Model file for the job. Use its own axes, mm. Face numbers are marked on the shaded views. A direction names the side the tool comes from. Round coordinates to 2 decimals unless told otherwise and drop trailing zeros. Loops run counter-clockwise (first coordinate to the right, second up) from the corner with the lowest first, then second, coordinate; pieces in that order, holes last. Notation, with made-up numbers: (2, 50) -> (20, 50) arc R34 cw to (20, 80) -> close; hole circle Ø6 at (37.25, 63.25). An arc over 180 degrees is marked (long way). Use a Markdown table: item, result.
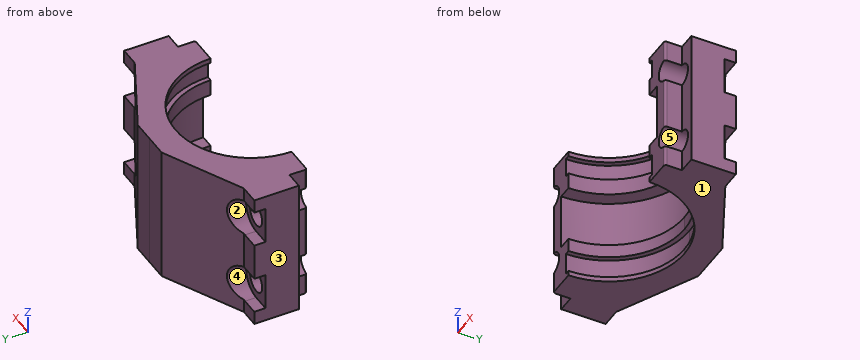
from build123d import *

# Parameters (mm, degrees)
BOSS_EXTRUDE1_DEPTH     = 56
SKETCH2_W               = 2
SKETCH2_H               = 7.81
SKETCH2_W_2             = 5.5
SKETCH2_H_2             = 23
SKETCH2_W_3             = 1.997029369
SKETCH2_H_3             = 9
CUT_EXTRUDE1_DEPTH      = 79.498407627
CUT_EXTRUDE1_DEPTH_BACK = 4.5
SKETCH5_R               = 4.5
CUT_EXTRUDE2_DEPTH      = 78.183223566


with BuildPart() as part:
    # Sketch1 → Boss-Extrude1 (new body)
    with BuildSketch(Plane.XY):
        with BuildLine():
            Line((-30.5, 0), (-41, 0))
            ThreePointArc((-41, 0), (-41.707106781, 0.292893219), (-42, 1))
            Line((-42, 1), (-42, 7))
            Line((-42, 7), (-49, 7))
            Line((-49, 7), (-49, 25))
            Line((-49, 25), (-41.09, 25))
            Line((-41.09, 25), (-9, 41))
            Line((-9, 41), (0, 41))
            Line((0, 41), (0, 30.5))
            ThreePointArc((0, 30.5), (-21.566756826, 21.566756826), (-30.5, 0))
        make_face()
    extrude(amount=-BOSS_EXTRUDE1_DEPTH)

    # Sketch2 → Cut-Revolve6 (revolve, cut)
    with BuildSketch(Plane.XZ):
        with Locations((-31.5, -5.905)):
            Rectangle(SKETCH2_W, SKETCH2_H)
        with Locations((-33.25, -28)):
            Rectangle(SKETCH2_W_2, SKETCH2_H_2)
        with Locations((-31.498514685, -49.5)):
            Rectangle(SKETCH2_W_3, SKETCH2_H_3)
    revolve(axis=Axis((0, 0, 0), (0, 0, -1)), mode=Mode.SUBTRACT)

    # Sketch4 → Cut-Extrude1 (cut, two sides: drawn at the far end of the back side and taken through both)
    with BuildSketch(Plane(origin=(0, 25, 0), x_dir=(1, 0, 0), z_dir=(0, 1, 0)).offset(-CUT_EXTRUDE1_DEPTH_BACK)):
        with BuildLine():
            Line((-49, 50.5), (-42, 50.5))
            ThreePointArc((-42, 50.5), (-34.5, 43), (-42, 35.5))
            Line((-42, 35.5), (-49, 35.5))
            Line((-49, 35.5), (-49, 50.5))
        make_face()
        with BuildLine():
            Line((-49, 20.5), (-42, 20.5))
            ThreePointArc((-42, 20.5), (-34.5, 13), (-42, 5.5))
            Line((-42, 5.5), (-49, 5.5))
            Line((-49, 5.5), (-49, 20.5))
        make_face()
    extrude(amount=CUT_EXTRUDE1_DEPTH + CUT_EXTRUDE1_DEPTH_BACK, mode=Mode.SUBTRACT)

    # Sketch5 → Cut-Extrude2 (cut, through all)
    with BuildSketch(Plane(origin=(0, 20.5, 0), x_dir=(1, 0, 0), z_dir=(0, 1, 0))):
        with Locations(Location((-42, 13, 0), (0, 0, 270))):
            Circle(SKETCH5_R)
        with Locations(Location((-42, 43, 0), (0, 0, 270))):
            Circle(SKETCH5_R)
    extrude(amount=-CUT_EXTRUDE2_DEPTH, mode=Mode.SUBTRACT)

    # Mirror1: part across plane


with BuildPart() as part_1:
    add(part.part)
    add(part.part.mirror(Plane(origin=(0, 41, -56), x_dir=(0, 0, 1), z_dir=(-1, 0, 0))))


solid = part_1.part
Q1. Band-saw the part on A-A, the plane z = -13. Give the cut face in (x, y), plus the area to 3 significant figures.
Results list:
| item | result |
|---|---|
| outline | (-49, 7) -> (-46.5, 7) -> (-46.5, 20.5) -> (-49, 20.5) -> close; (-37.5, 0) -> (-30.5, 0) arc R30.5 cw to (30.5, 0) -> (37.5, 0) -> (37.5, 20.5) -> (34.5, 20.5) -> (34.5, 28.29) -> (9, 41) -> (-9, 41) -> (-34.5, 28.29) -> (-34.5, 20.5) -> (-37.5, 20.5) -> close; (46.5, 7) -> (49, 7) -> (49, 20.5) -> (46.5, 20.5) -> close |
| area | 1,230 mm² |
Q2. Flat gauge pins, fed straight in: pin 1 (1.5 mm diameter, centred on y = 22.5, z = -39, fed in from +X); pin 2 (8 mm diameter, centred on x = 12, z = -13, fed in from -Y); pin 3 (5 mm diameter, centred on y = 29.5, z = -37, fed in from -X); pin 4 (6.5 mm diameter, centred on y = 4.5, z = -5, fed in from -X). Where does each tip first touch, or does it go through?
Results list:
| item | result |
|---|---|
| pin 1 | stops at x = 36.2 |
| pin 2 | stops at y = 25.97 |
| pin 3 | stops at x = -37.08 |
| pin 4 | stops at x = -49 |
Q3. Drill centre lines: L1, parallel to Z at x = -42, y = 13; L2, parallel to Z at x = -30.5, y = 3; L3, parallel to Z at x = 43, y = 9. Where is each one in solid material? Low to high. Write a range as from..to.
Results list:
| item | result |
|---|---|
| L1 | z = -56..-47.5, -38.5..-17.5, -8.5..0 |
| L2 | z = -56..-54, -45..-39.5, -16.5..-9.81, -2..0 |
| L3 | z = -56..-47.39, -38.61..-17.39, -8.61..0 |
Q4. Band-saw the part on D-D, the plane x = -23. Give the cut face in (y, z).
Results list:
| item | result |
|---|---|
| outline | (20.03, -56) -> (34.02, -56) -> (34.02, 0) -> (20.03, 0) -> (20.03, -2) -> (22.96, -2) -> (22.96, -9.81) -> (20.03, -9.81) -> (20.03, -16.5) -> (27.69, -16.5) -> (27.69, -39.5) -> (20.03, -39.5) -> (20.03, -45) -> (22.96, -45) -> (22.96, -54) -> (20.03, -54) -> close |
Q5. Pull direction Z, two halves, no side cores. Call the marked faces 1, 2 and 3: released by +Z, released by -Z, zero draft, split by the parting line, or undercut.
Results list:
| item | result |
|---|---|
| face 1 | released by -Z |
| face 2 | undercut |
| face 3 | zero draft |
Q6. Band-saw the part on C-C, the plane y = 11.5. Give the number of separate pieces and of enclosed holes in the cut face, plus the area to 3 significant figures.
Results list:
| item | result |
|---|---|
| separate pieces | 2 |
| enclosed holes | 4 |
| area | 1,730 mm² |
Q7. Band-saw the part on B-B, the plane z = -25. Give the cut face in (x, y).
Results list:
| item | result |
|---|---|
| outline | (-49, 7) -> (-42, 7) -> (-42, 1) arc R1 ccw to (-41, 0) -> (-36, 0) arc R36 cw to (36, 0) -> (41, 0) arc R1 ccw to (42, 1) -> (42, 7) -> (49, 7) -> (49, 25) -> (41.09, 25) -> (9, 41) -> (-9, 41) -> (-41.09, 25) -> (-49, 25) -> close |
Q8. Tool access for the marked faces 4 and 5: list every direction of +Z, -Z, +X, -X, +Y, -Y with a clear straight run to the whole face (end or side of a thin tool).
Results list:
| item | result |
|---|---|
| face 4 | -X, +Y |
| face 5 | +Y, -Y |
